Here's how the part is built. I have some questions about the finished solid (model axes, mm). Give positions to 0.01 mm unless a question says otherwise; leave off trailing zeros. Loops run counter-clockwise (first coordinate to the right, second up) from the corner with the lowest first, then second, coordinate; pieces in that order, holes last. Notation, with made-up numbers: (27, 76.5) - (64, 76.5) arc R16 ccw to (64, 82.5) - close; hole circle Ø2 at (-15.75, 69). An arc over 180 degrees is marked (long way). One line per item, written item: value. Start each with the question number.
```python
from build123d import *

# Parameters (mm, degrees)
SKETCH1_W           = 280.4
SKETCH1_H           = 12
BOSS_EXTRUDE1_DEPTH = 3
SKETCH3_R           = 1.5
CUT_EXTRUDE1_DEPTH  = 141.360393274
SKETCH6_W           = 140.2
SKETCH6_H           = 12
CUT_EXTRUDE2_DEPTH  = 141.360393274
SKETCH7_W           = 1.95
SKETCH7_H           = 1.95
CUT_EXTRUDE3_DEPTH  = 4
FILLET1_R           = 0.6


with BuildPart() as part:
    # Sketch1 → Boss-Extrude1 (new body)
    with BuildSketch(Plane(origin=(0, 0, 0), x_dir=(1, 0, 0), z_dir=(0, 1, 0))):
        Rectangle(SKETCH1_W, SKETCH1_H)
    extrude(amount=BOSS_EXTRUDE1_DEPTH)

    # Sketch3 → Cut-Extrude1 (cut, through all)
    with BuildSketch(Plane(origin=(0, 3, 0), x_dir=(1, 0, 0), z_dir=(0, 1, 0))):
        with Locations(Location((-136.25, 0, 0), (0, 0, 270))):
            Circle(SKETCH3_R)
        with Locations(Location((136.25, 0, 0), (0, 0, 270))):
            Circle(SKETCH3_R)
    extrude(amount=-CUT_EXTRUDE1_DEPTH, mode=Mode.SUBTRACT)

    # Sketch6 → Cut-Extrude2 (cut, through all)
    with BuildSketch(Plane(origin=(0, 3, 0), x_dir=(1, 0, 0), z_dir=(0, 1, 0))):
        with Locations((-70.1, 0)):
            Rectangle(SKETCH6_W, SKETCH6_H)
    extrude(amount=-CUT_EXTRUDE2_DEPTH, mode=Mode.SUBTRACT)

    # Sketch7 → Cut-Extrude3 (cut)
    with BuildSketch(Plane.ZY):
        with Locations((0, 1.5)):
            Rectangle(SKETCH7_W, SKETCH7_H)
    extrude(amount=-CUT_EXTRUDE3_DEPTH, mode=Mode.SUBTRACT)

    # Fillet1
    fillet1_edges = [part.edges().sort_by_distance(p)[0] for p in [
        (4, 1.5, 0.975),
        (4, 0.525, 0),
        (4, 1.5, -0.975),
        (4, 2.475, 0),
    ]]
    fillet(fillet1_edges, radius=FILLET1_R)


solid = part.part
```
(1) If we mould it in two halves opening along X, with no side actions, what happens to faces 1 (the face through (137.737, 1.521, -0.195)), 2 (the face through (140.2, 1, 0)), 3 (the face through (69, 0, 0))? For each: pulls with the +X half, pulls with the -X half, needs draft (parallel to the pull), parting line crosses it, or undercut.
(2) If we section it at A-A on x = 136.25: List the corners of the cut face in (y, z) for me.
(3) Will this pin go through, and if not, where does the flat tip stop? pin 1 (2.5 mm diameter, centred on x = 136.25, z = 0, fed in from -Y).
(4) Please list where these lines run through material, in increasing order: probe 1 along Z at (x, y) = (136.25, 2.35); probe 2 along X at (y, z) = (1.6, 0); probe 3 along X at (y, z) = (0.8, 0). Write a range as from..to.
Found:
1. face 1: undercut
1. face 2: pulls with the +X half
1. face 3: needs draft
2. outline: (0, -6) - (3, -6) - (3, -1.5) - (0, -1.5) - close; (0, 1.5) - (3, 1.5) - (3, 6) - (0, 6) - close
3. pin 1: through
4. probe 1: -6..-1.5, 1.5..6
4. probe 2: 4..134.75, 137.75..140.2
4. probe 3: 3.9..134.75, 137.75..140.2
